Design review of the part built by this model. Coordinates are the model's own, in mm. A direction names the side the tool comes from. Coordinates: 2 decimals unless noted, no trailing zeros. Order: outer loops, then holes, each group sorted by start corner. A loop starts at its lowest first (then second) coordinate and runs counter-clockwise, first axis right, second up. Notation, with made-up numbers: (43.25, -40) -> (86.25, -40) arc R24 cw to (86.25, -30) -> close; hole circle Ø9 at (-7, 31). An arc over 180 degrees is marked (long way). Write item = value, one per line.
Autodesk Inventor part; units mm, degrees
ref_plane "YZ Plane" through (0, 0, 0) normal (1, 0, 0) x (0, 1, 0)
ref_plane "XZ Plane" through (0, 0, 0) normal (0, 1, 0) x (-1, 0, 0)
ref_plane "XY Plane" through (0, 0, 0) normal (0, 0, 1) x (1, 0, 0)
sketch "Sketch1" plane through (0, 0, 0) normal (0, 0, 1) x (1, 0, 0)
  line L0 (-43.75, 33) -> (43.75, 33)
  line L1 (43.75, 33) -> (43.75, -33)
  line L2 (43.75, -33) -> (-43.75, -33)
  line L3 (-43.75, -33) -> (-43.75, 33)
  point P0 (0, 0)
  point P1 (0, 33)
  point P2 (-43.75, 0)
  dimension "d0" = 87.5
  dimension "d1" = 66
extrude "Extrusion1" add sketch "Sketch1" along normal blind 8
sketch "Sketch4" plane through (0, 0, 8) normal (0, 0, 1) x (1, 0, 0)
  line L0 (43.75, 33) -> (-43.75, 33)
  line L1 (-43.75, 33) -> (-43.75, -33)
  circle A0 centre (-37.25, 24) radius 5.4
  circle A1 centre (-37.25, -24) radius 5.4
  line L2 (-43.75, -33) -> (43.75, -33)
  point P0 (0, 0)
  dimension "d27" = 6.5
  dimension "d28" = 9
  dimension "d29" = 10.8
  dimension "d30" = 9
extrude "Extrusion4" cut sketch "Sketch4" against normal through all
sketch "Sketch5" plane through (0, 0, 8) normal (0, 0, 1) x (1, 0, 0)
  circle A0 centre (-25.0012, 0) radius 4
  circle A1 centre (-25.0012, 0) radius 8
  line L0 (-43.75, 33) -> (-43.75, -33)
  line L1 (43.75, 33) -> (-43.75, 33)
  circle A2 centre (-25.0012, 0) radius 4
  circle A3 centre (-25.0012, 0) radius 7
  point P0 (0, 0)
  point P1 (-43.75, 0)
  dimension "d24" = 16
  dimension "d33" = 18.7488
extrude "Extrusion5" cut sketch "Sketch5" against normal through all contours A0 | A1 | A3
sketch "Sketch6" plane through (0, 0, 8) normal (0, 0, 1) x (1, 0, 0)
  circle A0 centre (-40.5012, 15.5) radius 1.75
  circle A1 centre (-9.5012, 15.5) radius 1.75
  circle A2 centre (-9.5012, -15.5) radius 1.75
  circle A3 centre (-40.5012, -15.5) radius 1.75
  line L0 (-40.5012, 15.5) -> (-9.5012, 15.5)
  line L1 (-9.5012, 15.5) -> (-9.5012, -15.5)
  line L2 (-9.5012, -15.5) -> (-40.5012, -15.5)
  line L3 (-40.5012, -15.5) -> (-40.5012, 15.5)
  line L4 (-40.5012, 15.5) -> (-9.5012, -15.5) construction
  line L5 (-9.5012, 15.5) -> (-40.5012, -15.5) construction
  circle A4 centre (-25.0012, 0) radius 8
  line L6 (-43.75, 33) -> (-43.75, -33)
  line L7 (43.75, 33) -> (-43.75, 33)
  circle A5 centre (-40.5012, -15.5) radius 2.75
  circle A6 centre (-9.5012, 15.5) radius 3
  point P0 (0, 0)
  point P1 (-25.0012, 0)
  dimension "d35" = 3.5
  dimension "d36" = 31
extrude "Extrusion6" cut sketch "Sketch6" against normal through all contours L0 L3 A0 | A0 L3 L0 | L0 L1 A1 | A1 L1 L0 | L3 L2 A3 | A3 L2 L3 | L1 L2 A2 | A2 L2 L1
sketch "Sketch8" plane through (0, 0, 0) normal (0, 0, -1) x (-1, 0, 0)
  line L0 (-43.75, 33) -> (43.75, 33)
  line L1 (-43.75, -33) -> (-43.75, 33)
  point P0 (0, 0)
  point P1 (-39.75, 28)
  point P2 (-39.75, 13)
  point P3 (-39.75, -13)
  point P4 (-39.75, -28)
  dimension "d38" = 5
  dimension "d39" = 15
  dimension "d40" = 26
  dimension "d41" = 15
  dimension "d42" = 4
hole "Hole1" at (39.75, 28, 0) direction (0, 0, 1) diameter 4 end through all
pattern_linear "Rectangular Pattern1" count 2 spacing 15 along (0, -1, 0) count 2 spacing 41 along (0, -1, 0) of "Hole1"
pattern_linear "Rectangular Pattern2" count 2 spacing 27 along (-1, 0, 0) of "Hole1", "Rectangular Pattern1"
sketch "Sketch9" plane through (-43.75, -33, 0) normal (0, -1, 0) x (1, 0, 0)
  line L0 (0, 0) -> (0, 8)
  point P0 (43.75, 0)
  point P1 (6.5, 4)
  point P2 (0, 4)
  dimension "d59" = 6.5
hole "Hole2" at (-37.25, -33, 4) direction (0, 1, 0) diameter 4.134 depth 7.45 tip angle 118
sketch "Sketch10" plane through (-43.75, 33, 0) normal (0, 1, 0) x (1, 0, 0)
  circle A0 centre (6.5, -4) radius 2.067
  point P0 (43.75, 0)
hole "Hole3" at (-37.25, 33, 4) direction (0, -1, 0) diameter 4.134 depth 7.45 tip angle 118
equation "\"d30\" = d28"
properties part number "0005-10-027 suport nema Z" material "Wood (Maple)"
(1) For L1, parallel to X at y = -15.5, z = 4; L2, parallel to Y at x = -38, z = 6; L3, parallel to Y at x = -10, z = 4, list the stretches that pass through material, from the lowest coordinate up.
Report:
L1 = -43.75 to -42.25, -38.75 to -11.25, -7.75 to 43.75
L2 = -33 to -29.35, -18.65 to 18.65, 29.35 to 33
L3 = -33 to -17.18, -13.82 to 13.82, 17.18 to 33
(2) For faces 5 (the cylindrical face through (-9.729, -13.765, 4.056)), 6 (the cylindrical face through (-36.46, -30.97, 2.09)), list the 3-axis set-ups (+Z, -Z, +X, -X, +Y, -Y) from which the entire face can be reached by the end or side of a thin tool; tool diameter is ignored.
Report:
face_5 = +Z, -Z
face_6 = -Y
(3) We need section C-C (z = 4). Give the number of separate pieces and of enclosed holes in the cut face, and give its area (3 significant figures).
Report:
separate_pieces = 1
enclosed_holes = 13
area = 5,220 mm²
(4) We need section D-D (y = 28). Write out the cut boundary in (x, z).
Report:
outline = (-43.75, 0) -> (-40.88, 0) -> (-40.88, 8) -> (-43.75, 8) -> close; (-33.62, 0) -> (10.75, 0) -> (10.75, 8) -> (-33.62, 8) -> close; (14.75, 0) -> (37.75, 0) -> (37.75, 8) -> (14.75, 8) -> close; (41.75, 0) -> (43.75, 0) -> (43.75, 8) -> (41.75, 8) -> close
(5) We need section A-A (y = 0). Write out the cut boundary in (x, z).
Report:
outline = (-43.75, 0) -> (-33, 0) -> (-33, 8) -> (-43.75, 8) -> close; (-17, 0) -> (43.75, 0) -> (43.75, 8) -> (-17, 8) -> close
(6) The part is to be moulded in two halves that separate along Z. For faces 1 (the flat face through (-1, 0, 0)), 2 (the cylindrical face through (-36.46, 30.97, 5.91)), 3 (the flat face through (-1, 0, 8)), 4 (the flat face through (43.75, 0, 4)), say which applies: released by +Z, released by -Z, zero draft, split by the parting line, or undercut.
Report:
face_1 = released by -Z
face_2 = undercut
face_3 = released by +Z
face_4 = zero draft
(7) Insertion check: pin 1 (2.5 mm diameter, centred on x = 12.75, y = 28, fed in from -Z). The pin has a flat end and moves straight along its axis. Give the tip position at first contact, or say it passes through.
Report:
pin_1 = through
(8) We need section B-B (x = -37.25). Write out the cut boundary in (y, z).
Report:
outline = (-33, 0) -> (-29.4, 0) -> (-29.4, 1.93) -> (-33, 1.93) -> close; (-33, 6.07) -> (-29.4, 6.07) -> (-29.4, 8) -> (-33, 8) -> close; (-18.6, 0) -> (18.6, 0) -> (18.6, 8) -> (-18.6, 8) -> close; (29.4, 0) -> (33, 0) -> (33, 1.93) -> (29.4, 1.93) -> close; (29.4, 6.07) -> (33, 6.07) -> (33, 8) -> (29.4, 8) -> close
